Source: CAD feature listing. Evaluate the final solid. Frame: model axes, mm. A direction names the side the tool comes from. Coordinates: 2 decimals unless noted, no trailing zeros. Write each loop counter-clockwise with the first axis right and the second up, starting at its lowest first coordinate (ties: lowest second). Pieces come first, ordered by that corner, then holes. Notation, with made-up numbers: (40.5, 27) - (57.5, 27) arc R22 ccw to (57.5, 56) - close; hole circle Ø4 at (-11, 75.25). An arc over 180 degrees is marked (long way). One line per item, written item: value.
from build123d import *

# Parameters (mm, degrees)
F0_W        = 75
F0_H        = 75
F1_DEPTH    = 3.5
F2_W        = 65
F2_H        = 65
F3_DEPTH    = 3.5
F4_R        = 5
F6_DEPTH    = 65
F7_T        = 3
F7_T3_DEPTH = 70.7303019134
F7_T5_DEPTH = 71
F7_T7_DEPTH = 6.5680995141
F7_T9_DEPTH = 6.5
F8_W        = 67
F8_H        = 67
F9_DEPTH    = 2
F10_R       = 5


# Not quite as in the source:
# - a shell that OpenCascade refuses in one call is made with other operations: the cavity is built on its own and cut out


with BuildPart() as f1:
    # F0 (on Top) → F1 (new body)
    with BuildSketch(Plane.XY):
        with Locations((1.4847200364, -1.2060580678)):
            Rectangle(F0_W, F0_H)
    extrude(amount=F1_DEPTH)

    # F2 (on face) → F3 (cut)
    with BuildSketch(Plane.XY.offset(3.5)):
        with Locations((1.4847200364, -1.2060580678)):
            Rectangle(F2_W, F2_H)
    extrude(amount=-F3_DEPTH, mode=Mode.SUBTRACT)

    # F4
    f4_edges = [f1.edges().sort_by_distance(p)[0] for p in [
        (38.98472, -38.706058, 1.75),
        (-36.01528, -38.706058, 1.75),
        (38.98472, 36.293942, 1.75),
        (-36.01528, 36.293942, 1.75),
    ]]
    fillet(f4_edges, radius=F4_R)

    # F5 (on face) → F6 (join)
    with BuildSketch(Plane(origin=(0, -33.7060580678, 0), x_dir=(-1, 0, 0), z_dir=(0, 1, 0))):
        Polygon((31.0152799636, 3.5), (-33.9847200364, 3.5), (-33.9847200364, -57), (0, -57), (31.0152799636, 0.5), align=None)
    extrude(amount=F6_DEPTH)

    # F7: shell of thickness 3, made by hand


with BuildPart() as f7_core1:
    # F7_t2: copy of F1
    add(f1.part)

    # the walls: a layer under each face that stays
    f7_faces = [f7_core1.faces().sort_by_distance(p)[0] for p in [
        (1.4847200364, 36.2939419322, 1.75),
        (-33.5152799636, -36.2060580678, 0),
        (37.5202539423, 34.8294758382, 1.75),
        (-34.5508138695, 34.8294758382, 1.75),
        (38.9847200364, -1.2060580678, 1.75),
        (-36.0152799636, -1.2060580678, 1.75),
        (37.5202539423, -37.2415919737, 1.75),
        (-34.5508138695, -37.2415919737, 1.75),
        (1.4847200364, -38.7060580678, 1.75),
        (-30.9703302825, -33.7060580678, 0.0833333333),
        (1.6195690797, -33.7060580678, -28.5),
        (33.9847200364, -1.2060580678, -28.5),
        (1.6195690797, 31.2939419322, -28.5),
        (-30.8804309203, 31.2939419322, 0.0833333333),
        (-31.0152799636, -1.2060580678, 0.25),
        (-15.5076399818, -1.2060580678, -28.25),
        (16.9923600182, -1.2060580678, -57),
    ]]
    thicken(f7_faces, amount=-F7_T, mode=Mode.SUBTRACT)

    # F7_s4 → F7_t3 (cut)
    with BuildSketch(Plane.YZ.offset(-33.745581877)):
        Polygon((-33.7360580678, -0.03), (-33.7060580678, 3), (-30.7060580678, 3), (-30.7060580678, 0), align=None)
        Polygon((31.3239419322, -0.03), (31.2939419322, 3), (28.2939419322, 3), (28.2939419322, 0), align=None)
    extrude(amount=F7_T3_DEPTH, mode=Mode.SUBTRACT)

    # F7_s6 → F7_t5 (cut)
    with BuildSketch(Plane.XZ.offset(-34.2939419322)):
        Polygon((34.0147200364, -0.03), (33.9847200364, 3), (30.9847200364, 3), (30.9847200364, 0), align=None)
        Polygon((-31.0116837883, 0.485757878), (-34.0152799636, 0.5), (-34.0152799636, 12.3810577497), (-28.3748974906, 1.9242122019), align=None)
    extrude(amount=F7_T5_DEPTH, mode=Mode.SUBTRACT)

    # F7_s8 → F7_t7 (cut)
    with BuildSketch(Plane(origin=(-5.5050917478, 0, 10.2060267027), x_dir=(0, 1, 0), z_dir=(-0.4747374006, 0, 0.880127491))):
        Polygon((-33.6760580678, 27.0900318369), (-36.7060580678, 27.0600318369), (-36.7060580678, 24.0600318369), (-33.7060580678, 24.0600318369), align=None)
        Polygon((31.2639419322, 27.0900318369), (34.2939419322, 27.0600318369), (34.2939419322, 24.0600318369), (31.2939419322, 24.0600318369), align=None)
    extrude(amount=F7_T7_DEPTH, mode=Mode.SUBTRACT)

    # F7_s10 → F7_t9 (cut)
    with BuildSketch(Plane.XY.offset(-3)):
        Polygon((-30.9852799636, -33.6760580678), (-31.0152799636, -36.7060580678), (-34.0152799636, -36.7060580678), (-34.0152799636, -33.7060580678), align=None)
        Polygon((-30.9852799636, 31.2639419322), (-31.0152799636, 34.2939419322), (-34.0152799636, 34.2939419322), (-34.0152799636, 31.2939419322), align=None)
    extrude(amount=F7_T9_DEPTH, mode=Mode.SUBTRACT)


with BuildPart() as f1_1:
    add(f1.part)

    # what is left inside the walls is the cavity
    f7_cavity = [f7_core1.part.solids().sort_by_distance(p)[0] for p in [
        (3.379924, -12.706058, 3.47),
    ]]
    add(f7_cavity, mode=Mode.SUBTRACT)

    # F8 (on face) → F9 (cut)
    with BuildSketch(Plane.XY.offset(3.5)):
        with Locations((1.4847200364, -1.2060580678)):
            Rectangle(F8_W, F8_H)
    extrude(amount=-F9_DEPTH, mode=Mode.SUBTRACT)

    # F10
    f10_edges = [f1_1.edges().sort_by_distance(p)[0] for p in [
        (-32.01528, 32.293942, 2.5),
        (34.98472, 32.293942, 2.25),
        (-32.01528, -34.706058, 2.5),
        (34.98472, -34.706058, 2.25),
    ]]
    fillet(f10_edges, radius=F10_R)


solid = f1_1.part
1) Section query B-B on x = 20.5. Output: boundary loops of the cut face in (y, z).
Values found:
outline: (-38.71, 0) - (-33.71, 0) - (-33.71, -57) - (31.29, -57) - (31.29, 0) - (36.29, 0) - (36.29, 3.5) - (33.29, 3.5) - (33.29, 3) - (32.29, 3) - (32.29, 1.5) - (28.29, 1.5) - (28.29, -54) - (-30.71, -54) - (-30.71, 1.5) - (-34.71, 1.5) - (-34.71, 3) - (-35.71, 3) - (-35.71, 3.5) - (-38.71, 3.5) - close
2) Reachability of faces 4 (the flat face through (-36.015, -2, 2)), 5 (the flat face through (-12.968, -1.619, -26.638)) from +Z, -Z, +X, -X, +Y, -Y: full face, straight path, thin tool, end or side. Return the list, or none.
Values found:
face 4: +Z, -Z, -X, +Y, -Y
face 5: +Z
3) Contact query for flat-ended pins moving along their axis: P1, Ø20, axis at x = -0.5, y = 6.5, coming from the +Z side; P2, Ø1.5, axis at x = -1, z = -31, coming from the -Y side; P3, Ø3, axis at y = 20.5, z = -36.5, coming from the -X side. Output: stop coordinate, or through.
Values found:
P1: z = -31.21
P2: y = -33.71
P3: x = -11.87
4) Section query C-C on z = -49. Output: boundary loops of the cut face in (x, y).
Values found:
outline: (-4.32, -33.71) - (33.98, -33.71) - (33.98, 31.29) - (-4.32, 31.29) - close; hole (-0.91, -30.71) - (30.98, -30.71) - (30.98, 28.29) - (-0.91, 28.29) - close
5) Section query A-A on y = -6.5. Output: boundary loops of the cut face in (x, z).
Values found:
outline: (-36.02, 0) - (-31.02, 0) - (-31.02, 0.5) - (0, -57) - (33.98, -57) - (33.98, 0) - (38.98, 0) - (38.98, 3.5) - (35.98, 3.5) - (35.98, 3) - (34.98, 3) - (34.98, 1.5) - (30.98, 1.5) - (30.98, -54) - (1.79, -54) - (-28.15, 1.5) - (-32.02, 1.5) - (-32.02, 3.5) - (-36.02, 3.5) - close
6) Draft query along X for faces 1 (the flat face through (8, 28.294, -26)), 2 (the flat face through (33.985, -2, -28)), 3 (the cylindrical face through (-34.59, 34.79, 1.77)). Return one class per face: released by +X, released by -X, zero draft, split by the parting line, or undercut.
Values found:
face 1: undercut
face 2: released by +X
face 3: released by -X
7) Section query D-D on z = -30.5. Output: boundary loops of the cut face in (x, y), then the cut area to 3 significant figures.
Values found:
outline: (-14.29, -33.71) - (33.98, -33.71) - (33.98, 31.29) - (-14.29, 31.29) - close; hole (-10.89, -30.71) - (30.98, -30.71) - (30.98, 28.29) - (-10.89, 28.29) - close
area: 668 mm2
8) Material intervals for line 1 (Y direction, x = -2, z = -12); line 2 (Z direction, x = 10, y = 9.5); line 3 (Z direction, x = 32.5, y = -34.5), sorted ascending.
Values found:
line 1: -33.71 to -30.71, 28.29 to 31.29
line 2: -57 to -54
line 3: 0 to 3
